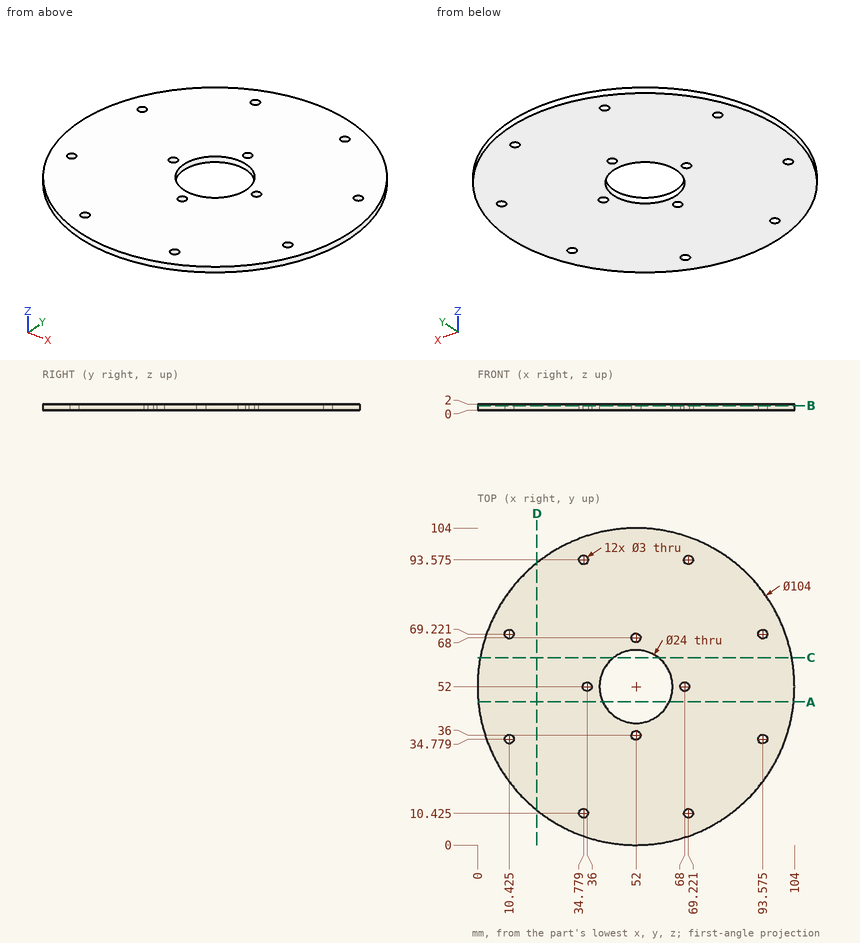
Print and shaded views of the part. All mm, measured from the part's lowest x, y and z. Coordinates: 2 decimals unless noted, no trailing zeros. Loops run counter-clockwise (first coordinate to the right, second up) from the corner with the lowest first, then second, coordinate; pieces in that order, holes last. Notation, with made-up numbers: (-16, 37.25) - (30, 37.25) arc R26 ccw to (30, 58.25) - close; hole circle Ø11 at (58.5, 62.5). An arc over 180 degrees is marked (long way). Write item = value, one per line. Start each with the question number.
Item 1: Wall check: L1, parallel to Y at x = 52, z = 0.55; L2, parallel to Y at x = 93, z = 1.35 (1 decimal); L3, parallel to X at y = 51, z = 1.2. Give the ranges that are in metal, low to high. Write a range as from..to.
Item 2: Flat gauge pin, fed straight in: pin 1 Ø3.5 at (x, y) = (69.22, 10.43) entering from -Z. Where does the tip first touch, or does it go through?
Item 3: Cut at A-A, the plane y = 47. Give the cut face in (x, z).
Item 4: Cut at D-D, the plane x = 19.5. Give the cut face in (y, z).
Item 5: Cut at B-B, the plane z = 1.5. State how many separate pieces and enclosed holes the cut face has, and give its area (3 significant figures).
Item 6: Cut at C-C, the plane y = 61.5. Give the cut face in (x, z) (1 decimal), and give its area (3 significant figures).
The answers:
q1.L1 = 0..34.5, 37.5..40, 64..66.5, 69.5..104
q1.L2 = 20..33.4, 36.2..67.8, 70.6..84
q1.L3 = 0.01..34.88, 37.12..40.04, 63.96..66.88, 69.12..103.99
q2.pin_1 = 0
q3.outline = (0.24, 0) - (41.09, 0) - (41.09, 2) - (0.24, 2) - close; (62.91, 0) - (103.76, 0) - (103.76, 2) - (62.91, 2) - close
q4.outline = (11.41, 0) - (92.59, 0) - (92.59, 2) - (11.41, 2) - close
q5.separate_pieces = 1
q5.enclosed_holes = 13
q5.area = 7,960 mm2
q6.outline = (0.9, 0) - (44.7, 0) - (44.7, 2) - (0.9, 2) - close; (59.3, 0) - (103.1, 0) - (103.1, 2) - (59.3, 2) - close
q6.area = 175 mm2
